Input: dimensioned drawing with shaded views. Units: mm. Origin: part minimum x, y, z. A direction names the side the tool comes from. Give positions to 0.01 mm unless a question says otherwise; leave off trailing zeros. Loops run counter-clockwise (first coordinate to the right, second up) from the corner with the lowest first, then second, coordinate; pieces in that order, holes last.
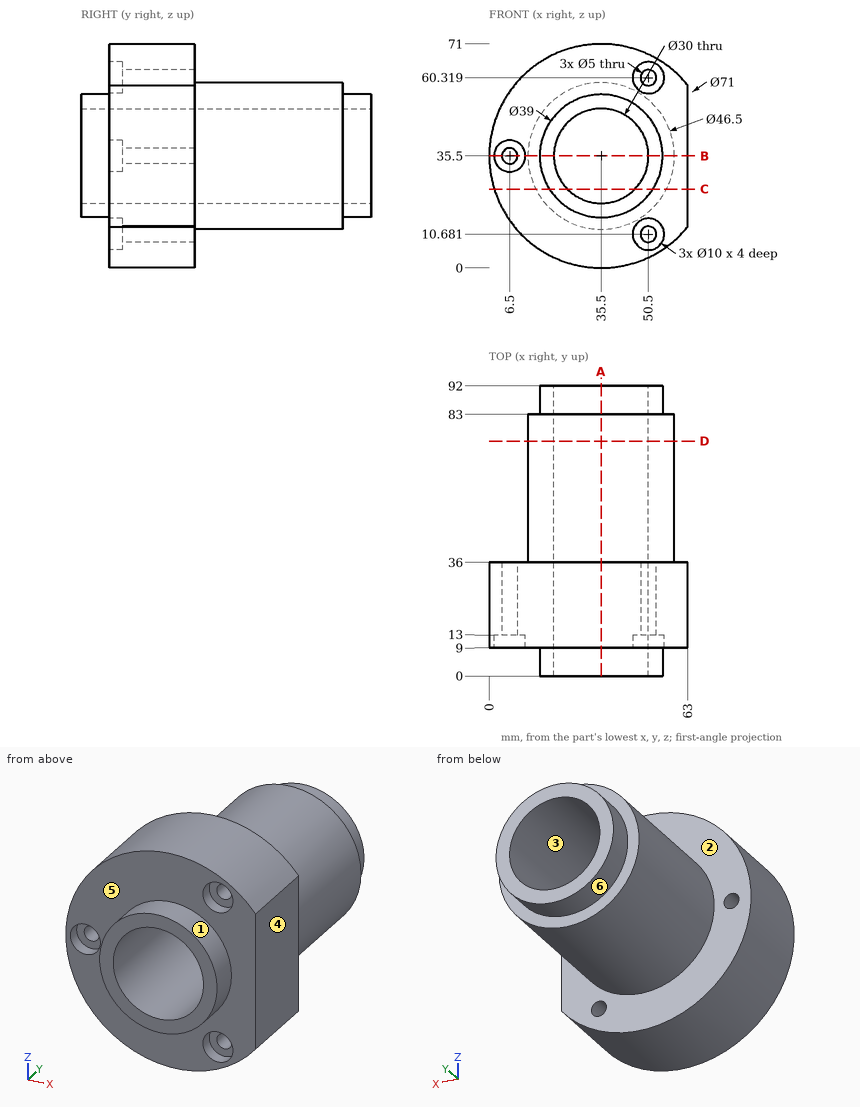
(1) Section D-D, the plane y = 74.5. Return the cut outline in (x, z).
A:
outline: circle Ø46.5 at (35.5, 35.5); hole circle Ø30 at (35.5, 35.5)
(2) Mould query, pull axis X, two halves, no side actions, for the marked faces 1, 2 and 3. Classes: pulls with the +X half, pulls with the -X half, needs draft (parallel to the pull), parting line crosses it, or undercut.
A:
face 1: parting line crosses it
face 2: needs draft
face 3: undercut
(3) Section A-A, the plane x = 35.5. Return the cut outline in (y, z).
A:
outline: (0, 16) - (9, 16) - (9, 0) - (36, 0) - (36, 12.25) - (83, 12.25) - (83, 16) - (92, 16) - (92, 20.5) - (0, 20.5) - close; (0, 50.5) - (92, 50.5) - (92, 55) - (83, 55) - (83, 58.75) - (36, 58.75) - (36, 71) - (9, 71) - (9, 55) - (0, 55) - close
(4) First-contact query: pin 1 (4.5 mm diameter, centred on x = 6.5, z = 35.5, fed in from +Y); pin 2 (11 mm diameter, centred on x = 5.5, z = 33, fed in from -Y); pin 3 (3 mm diameter, centred on y = 24, z = 45, fed in from -X); pin 4 (3 mm diameter, centred on x = 54, z = 54.5, fed in from +Y). Flat tips, straight axial feed; report the tip coordinate or a pass-through.
A:
pin 1: passes through
pin 2: stops at y = 9
pin 3: stops at x = 0.91
pin 4: stops at y = 36
(5) Section B-B, the plane z = 35.5. Return the cut outline in (x, y).
A:
outline: (0, 9) - (1.5, 9) - (1.5, 13) - (4, 13) - (4, 36) - (0, 36) - close; (9, 13) - (11.5, 13) - (11.5, 9) - (16, 9) - (16, 0) - (20.5, 0) - (20.5, 92) - (16, 92) - (16, 83) - (12.25, 83) - (12.25, 36) - (9, 36) - close; (50.5, 0) - (55, 0) - (55, 9) - (63, 9) - (63, 36) - (58.75, 36) - (58.75, 83) - (55, 83) - (55, 92) - (50.5, 92) - close
(6) Section C-C, the plane z = 25. Return the cut outline in (x, y), then the cut area to 3 significant figures.
A:
outline: (1.59, 9) - (19.07, 9) - (19.07, 0) - (24.79, 0) - (24.79, 92) - (19.07, 92) - (19.07, 83) - (14.76, 83) - (14.76, 36) - (1.59, 36) - close; (46.21, 0) - (51.93, 0) - (51.93, 9) - (63, 9) - (63, 36) - (56.24, 36) - (56.24, 83) - (51.93, 83) - (51.93, 92) - (46.21, 92) - close
area: 2,230 mm2
(7) Ray query, line 1 along X through (y, z) = (27.25, 35.5); line 2 along X through (y, z) = (12.25, 35.5); line 3 along Z through (x, y) = (35.5, 63). Return the intervals inside material, ascending.
A:
line 1: x = 0 to 4, 9 to 20.5, 50.5 to 63
line 2: x = 0 to 1.5, 11.5 to 20.5, 50.5 to 63
line 3: z = 12.25 to 20.5, 50.5 to 58.75
(8) Reachability of the marked faces 4, 5 and 6 from +Z, -Z, +X, -X, +Y, -Y: full face, straight path, thin tool, end or side. Return the list, or none.
A:
face 4: +Z, -Z, +X, +Y, -Y
face 5: -Y
face 6: +Y
